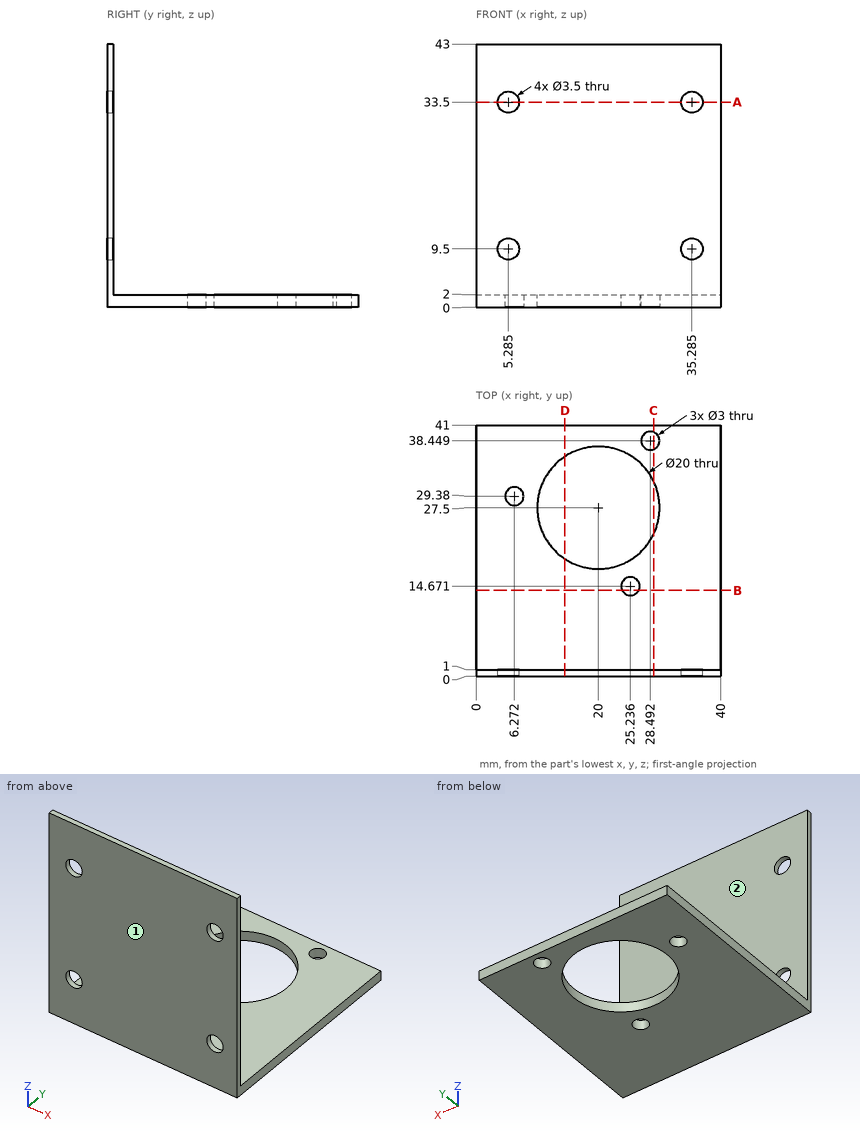
Job drawing, mm, ordinate dimensions from the low corner. One solid piece. A direction names the side the tool comes from. Round coordinates to 2 decimals unless told otherwise and drop trailing zeros. Loops run counter-clockwise (first coordinate to the right, second up) from the corner with the lowest first, then second, coordinate; pieces in that order, holes last. Notation, with made-up numbers: M 53.25,23.5 L 104.25,23.5 A21 ccw 104.25,34.5 Z; hole C 37.5,55.5 d8. An arc over 180 degrees is marked long. One line per question, with ' | ' between items. Start each with the question number.
Item 1: Cut at A-A, the plane z = 33.5. Write the cut outline in (x, y) (1 decimal).
Item 2: Cut at D-D, the plane x = 14.5. Write the cut outline in (y, z).
Item 3: Wall check: line 1 (X direction, y = 0.25, z = 33.5) (1 decimal); line 2 (Y direction, x = 25, z = 27); line 3 (Z direction, x = 29, y = 35). Give the ranges that are in metal, low to high.
Item 4: Which spindle directions (+Z, -Z, +X, -X, +Y, -Y) get a long thin tool onto all of the face, cutting with end or side? Do the marked faces 1 and 2. Say none if no direction does.
Item 5: Cut at B-B, the plane y = 14. Write the cut outline in (x, z) (1 decimal).
Item 6: Pin check, flat tips, straight feed: pin 1 Ø5.5 at (x, z) = (5.28, 9.5) entering from -Y; pin 2 Ø3 at (x, z) = (30, 23.5) entering from +Y; pin 3 Ø2 at (x, y) = (32.5, 33.5) entering from +Z. Stop position of each tip, or through.
Item 7: Cut at C-C, the plane x = 29. Write the cut outline in (y, z).
Responses:
1) outline: M 0,0 L 3.5,0 L 3.5,1 L 0,1 Z; M 7,0 L 33.5,0 L 33.5,1 L 7,1 Z; M 37,0 L 40,0 L 40,1 L 37,1 Z
2) outline: M 0,0 L 19.15,0 L 19.15,2 L 1,2 L 1,43 L 0,43 Z; M 35.85,0 L 41,0 L 41,2 L 35.85,2 Z
3) line 1: x = 0 to 3.5, 7 to 33.5, 37 to 40 | line 2: y = 0 to 1 | line 3: z = 0 to 2
4) face 1: +Z, -Z, +X, -X, -Y | face 2: +Z, +X, -X, +Y
5) outline: M 0,0 L 23.9,0 L 23.9,2 L 0,2 Z; M 26.6,0 L 40,0 L 40,2 L 26.6,2 Z
6) pin 1: stops at y = 0 | pin 2: stops at y = 1 | pin 3: stops at z = 2
7) outline: M 0,0 L 23.14,0 L 23.14,2 L 1,2 L 1,43 L 0,43 Z; M 31.86,0 L 37.04,0 L 37.04,2 L 31.86,2 Z; M 39.86,0 L 41,0 L 41,2 L 39.86,2 Z
